Autodesk Inventor part; units mm, degrees
ref_plane "YZ Plane" through (0, 0, 0) normal (1, 0, 0) x (0, 1, 0)
ref_plane "XZ Plane" through (0, 0, 0) normal (0, 1, 0) x (-1, 0, 0)
ref_plane "XY Plane" through (0, 0, 0) normal (0, 0, 1) x (1, 0, 0)
sketch "Sketch2" plane through (0, 0, 0) normal (1, 0, 0) x (0, 1, 0)
  circle A0 centre (0, 0) radius 45
  dimension "d7" = 90
extrude "Extrusion1" add sketch "Sketch2" along normal blind 5.588
sketch "Sketch3" plane through (5.588, 0, 0) normal (1, 0, 0) x (0, 0, -1)
  circle A0 centre (0, 0) radius 45
  line L0 (0, 0) -> (-45, 0)
  circle A1 centre (0, 0) radius 45
  point P0 (-40.325, 0)
  dimension "d10" = 40.325
hole "Hole1" at (5.588, 0, 40.325) direction (-1, 0, 0) diameter 3.1 end through all
pattern_circular "Circular Pattern1" count 40 over 360 about axis through (-10, 0, 0) along (1, 0, 0) of "Hole1"
sketch "Sketch4" plane through (5.588, 0, 0) normal (1, 0, 0) x (0, 0, -1)
  point P0 (0, 0)
  point P1 (0, 0)
hole "Hole2" at (5.588, 0, 0) direction (-1, 0, 0) diameter 20 end through all
sketch "Sketch5" plane through (5.588, 0, 0) normal (1, 0, 0) x (0, 0, -1)
  line L0 (0, -2.5) -> (-15, -2.5)
  line L1 (-15, -2.5) -> (-15, 2.5)
  line L2 (-15, 2.5) -> (0, 2.5)
  line L3 (0, 2.5) -> (0, -2.5)
  line L4 (-2.5, 0) -> (2.5, 0)
  line L5 (2.5, 0) -> (2.5, 15)
  line L6 (2.5, 15) -> (-2.5, 15)
  line L7 (-2.5, 15) -> (-2.5, 0)
  arc A0 (-15, 2.5) -> (-15, -2.5) centre (-15, 0) ccw
  arc A1 (2.5, 15) -> (-2.5, 15) centre (0, 15) ccw
  point P0 (0, 0)
  point P1 (0, 0)
  dimension "d28" = 5
  dimension "d29" = 5
  dimension "d30" = 15
  dimension "d31" = 15
extrude "Extrusion2" cut sketch "Sketch5" against normal through all
equation "\"d7\" = spoolDiameter"
equation "\"d8\" = spoolThickness"
equation "\"materialThickness\" = 3.175"
equation "\"laserKerf\" = 0.12"
equation "\"cardPinDiameter\" = 3"
equation "\"spoolDiameter\" = 90"
equation "\"centeralShaftDiameter\" = 8"
equation "\"cardHeight\" = 53.98"
equation "\"cardWidth\" = 85.6"
equation "\"cardThickness\" = 0.76"
equation "\"cardFillet\" = 2.88"
equation "\"cardClearence\" = 0.5"
equation "\"bearingOd\" = 22"
equation "\"bearingWidth\" = 8"
equation "\"axleHeight\" = 95"
equation "\"nutTrapDepth\" = 2.5"
equation "\"nutTrapwidth\" = 5.5"
equation "\"nutTrapClearence\" = 2"
equation "\"magnetDiameter\" = 6"
equation "\"magnetLength\" = 3"
equation "\"magnetProtusion\" = 0.25"
equation "\"spoolThickness\" = 5.588"
properties part number "spoolGearSide" material "Polycarbonate, Clear"
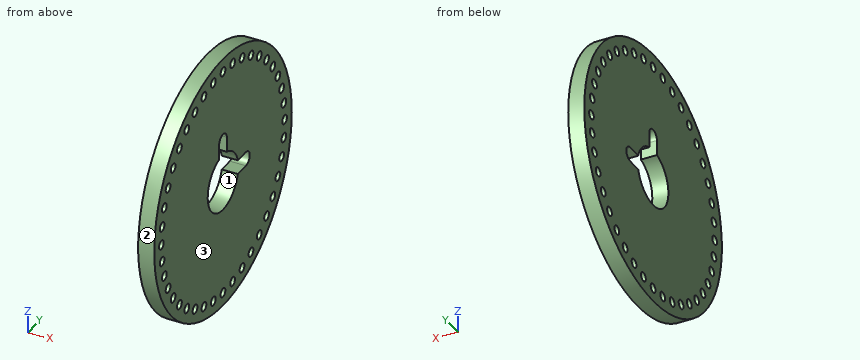
CAD build for the part. Positions are in the model's coordinates, mm. Face numbers are marked on the shaded views. Round coordinates to 2 decimals unless told otherwise and drop trailing zeros. Write each loop counter-clockwise with the first axis right and the second up, starting at its lowest first coordinate (ties: lowest second). Pieces come first, ordered by that corner, then holes. Notation, with made-up numbers: (46, 77) -> (71, 77) arc R32 cw to (71, 114) -> close; hole circle Ø9 at (-33, -12). An arc over 180 degrees is marked (long way). Answer in a Markdown table with one row per item. Add a question column.
Item 1: Saw through at A-A, the plane z = 0. Write the cut outline in (x, y) (3 decimals), then the cut area to 3 significant figures.
Item 2: Mould opens along Y. For the marked faces 1, 2 and 3 say: pulls with the +Y half, pulls with the -Y half, needs draft (parallel to the pull), parting line crosses it, or undercut.
Item 3: Drop flat-ended pins along their axis: pin 1 Ø1.9 at (y, z) = (-18.31, -35.93) entering from -X; pin 2 Ø3 at (x, y) = (1.5, 26) entering from +Z; pin 3 Ø1 at (x, y) = (3.5, 26) entering from +Z; pin 4 Ø3 at (x, z) = (3.5, 5.5) entering from +Y. Give the stop position or say it passes through.
Item 4: Drill centre lines: line 1 (Z direction, x = 3.1, y = -29); line 2 (Z direction, x = 4.85, y = 38); line 3 (Y direction, x = 4.5, z = 24.5). Where is each one in solid material? Low to high. Write a range as from..to.
Item 5: Saw through at D-D, the plane y = 33. Write the cut outline in (x, z), then the cut area to 3 significant figures.
Findings below:
| question | item | result |
|---|---|---|
| 1 | outline | (0, -45) -> (5.588, -45) -> (5.588, -41.875) -> (0, -41.875) -> close; (0, -38.775) -> (5.588, -38.775) -> (5.588, -10) -> (0, -10) -> close; (0, 17.5) -> (5.588, 17.5) -> (5.588, 38.775) -> (0, 38.775) -> close; (0, 41.875) -> (5.588, 41.875) -> (5.588, 45) -> (0, 45) -> close |
| 1 | area | 315 mm^2 |
| 2 | face 1 | undercut |
| 2 | face 2 | parting line crosses it |
| 2 | face 3 | needs draft |
| 3 | pin 1 | passes through |
| 3 | pin 2 | stops at z = 37.75 |
| 3 | pin 3 | stops at z = 37.08 |
| 3 | pin 4 | stops at y = 44.82 |
| 4 | line 1 | z = -34.41..-29.99, -27.04..27.04, 29.99..34.41 |
| 4 | line 2 | z = -24.1..-13.97, -10.95..10.95, 13.97..24.1 |
| 4 | line 3 | y = -37.75..-33.95, -31.29..31.29, 33.95..37.75 |
| 5 | outline | (0, -30.59) -> (5.59, -30.59) -> (5.59, -25.21) -> (0, -25.21) -> close; (0, -22.2) -> (5.59, -22.2) -> (5.59, 22.2) -> (0, 22.2) -> close; (0, 25.21) -> (5.59, 25.21) -> (5.59, 30.59) -> (0, 30.59) -> close |
| 5 | area | 308 mm^2 |
